The listing builds one solid part. Answer for the finished solid, in the listing's coordinates (mm). A direction names the side the tool comes from. Round coordinates to 2 decimals unless told otherwise and drop trailing zeros. Order: outer loops, then holes, each group sorted by start corner. A loop starts at its lowest first (then second) coordinate and runs counter-clockwise, first axis right, second up. Notation, with made-up numbers: M -24,46 L -5,46 A29 ccw -5,77 Z; hole C 55.25,50 d3. An arc over 180 degrees is marked long. Put each result on its own line as item: value. Start each with the question number.
1. Consider line 1 (Y direction, x = -1, z = 2.1); line 2 (Y direction, x = -0.5, z = 0.35); line 3 (X direction, y = -3, z = 2). Determine where each line is inside the solid, lowest interval first.
2. Which of the six approach directions +Z, -Z, +X, -X, +Y, -Y give full straight-line access (tool end or side, diameter ignored) to faces 4 (the face through (5.068, -39.625, 1.479)), 5 (the face through (-5.068, 39.625, 1.479)), 6 (the face through (-7.784, -38.298, 1.479))?
3. The part is cut by section B-B (x = 4.25). Give the vertices of the cut face in (y, z).
4. The part is cut by section D-D (y = -1.5). Give the vertices of the cut face in (x, z).
5. The part is cut by section A-A (y = 25). Give the vertices of the cut face in (x, z), then the cut area to 3 significant figures.
6. The mould has two halves that part along X. Classify faces 1 (the face through (13.386, -23.246, 1.479)), 2 (the face through (-5.124, -39.667, 1.479)), 3 (the face through (-7, -9, 3)): +X half, -X half, draft (parallel to the pull), parting line (faces both ways), or undercut.
7. The part is cut by section C-C (z = 0.75). Give the vertices of the cut face in (x, y), then the cut area to 3 significant figures.
8. Each of these flat-tipped pins is pushed along its axis until it touches: pin 1 Ø12 at (x, y) = (0, 3.5) entering from -Z; pin 2 Ø1 at (x, y) = (-7.5, -7.5) entering from -Z. Where does it stop, or does it pass through?
from build123d import *

# Parameters (mm, degrees)
F0_R     = 11
F1_DEPTH = 3


with BuildPart() as f1:
    # F0 (on Top) → F1 (new body)
    with BuildSketch(Plane.XY):
        with BuildLine():
            ThreePointArc((8.457802, -35.522148), (13.35858, -23.05107), (5.09902, -12.5))
            ThreePointArc((5.09902, -12.5), (13.5, 0), (5.09902, 12.5))
            ThreePointArc((5.09902, 12.5), (13.35858, 23.05107), (8.457802, 35.522148))
            Line((8.457802, 35.522148), (7.091197, 41.152409))
            Line((7.091197, 41.152409), (3.101335, 38.138939))
            Line((3.101335, 38.138939), (0, 42.245135))
            Line((0, 42.245135), (-3.101335, 38.138939))
            Line((-3.101335, 38.138939), (-7.091197, 41.152409))
            Line((-7.091197, 41.152409), (-8.457802, 35.522148))
            ThreePointArc((-8.457802, 35.522148), (-13.35858, 23.05107), (-5.09902, 12.5))
            ThreePointArc((-5.09902, 12.5), (-13.5, 0), (-5.09902, -12.5))
            ThreePointArc((-5.09902, -12.5), (-13.35858, -23.05107), (-8.457802, -35.522148))
            Line((-8.457802, -35.522148), (-7.091197, -41.152409))
            Line((-7.091197, -41.152409), (-3.101335, -38.138939))
            Line((-3.101335, -38.138939), (0, -42.245135))
            Line((0, -42.245135), (3.101335, -38.138939))
            Line((3.101335, -38.138939), (7.091197, -41.152409))
            Line((7.091197, -41.152409), (8.457802, -35.522148))
        make_face()
        with Locations((0, -25)):
            Circle(F0_R, mode=Mode.SUBTRACT)
        Circle(F0_R, mode=Mode.SUBTRACT)
        with Locations((0, 25)):
            Circle(F0_R, mode=Mode.SUBTRACT)
    extrude(amount=F1_DEPTH)


solid = f1.part
Resolved:
1. line 1: -40.92 to -35.95, -14.05 to -10.95, 10.95 to 14.05, 35.95 to 40.92
1. line 2: -41.58 to -35.99, -14.01 to -10.99, 10.99 to 14.01, 35.99 to 41.58
1. line 3: -13.16 to -10.58, 10.58 to 13.16
2. face 4: +Z, -Z, -Y
2. face 5: +Z, -Z, +Y
2. face 6: +Z, -Z, -X, -Y
3. outline: M -39.01,0 L -35.15,0 L -35.15,3 L -39.01,3 Z; M -14.85,0 L -10.15,0 L -10.15,3 L -14.85,3 Z; M 10.15,0 L 14.85,0 L 14.85,3 L 10.15,3 Z; M 35.15,0 L 39.01,0 L 39.01,3 L 35.15,3 Z
4. outline: M -13.42,0 L -10.9,0 L -10.9,3 L -13.42,3 Z; M 10.9,0 L 13.42,0 L 13.42,3 L 10.9,3 Z
5. outline: M -13.5,0 L -11,0 L -11,3 L -13.5,3 Z; M 11,0 L 13.5,0 L 13.5,3 L 11,3 Z
5. area: 15.0 mm2
6. face 1: +X half
6. face 2: undercut
6. face 3: draft
7. outline: M -8.46,-35.52 L -7.09,-41.15 L -3.1,-38.14 L 0,-42.25 L 3.1,-38.14 L 7.09,-41.15 L 8.46,-35.52 A13.5 ccw 5.1,-12.5 A13.5 ccw 5.1,12.5 A13.5 ccw 8.46,35.52 L 7.09,41.15 L 3.1,38.14 L 0,42.25 L -3.1,38.14 L -7.09,41.15 L -8.46,35.52 A13.5 ccw -5.1,12.5 A13.5 ccw -5.1,-12.5 A13.5 ccw Z; hole C 0,-25 d22; hole C 0,0 d22; hole C 0,25 d22
7. area: 620 mm2
8. pin 1: through
8. pin 2: z = 0
